Autodesk Inventor part; units mm, degrees
ref_plane "YZ Plane" through (0, 0, 0) normal (1, 0, 0) x (0, 1, 0)
ref_plane "XZ Plane" through (0, 0, 0) normal (0, 1, 0) x (-1, 0, 0)
ref_plane "XY Plane" through (0, 0, 0) normal (0, 0, 1) x (1, 0, 0)
sketch "Sketch2" plane through (0, 0, 0) normal (0, 0, 1) x (1, 0, 0)
  line L0 (0, 0) -> (87.9881, 0) construction
  line L1 (0, 0) -> (65.9905, 38.1011) construction
  line L2 (65.9905, 38.1011) -> (87.9881, 0) construction
  circle A0 centre (0, 0) radius 76.2 construction
  line L3 (62.5859, 43.4678) -> (34.9256, 27.4975)
  line L4 (68.9361, 32.4694) -> (41.2758, 16.4991)
  arc A1 (34.9256, 27.4975) -> (41.2758, 16.4991) centre (38.1007, 21.9983) ccw
  arc A2 (73.4536, 20.2735) -> (73.4536, -20.2735) centre (87.9881, 0) ccw
  arc A3 (73.4536, 20.2735) -> (68.9361, 32.4694) centre (0, 0) ccw
  line L5 (62.5873, -43.4657) -> (34.9265, -27.4963)
  arc A4 (41.2764, -16.4977) -> (34.9265, -27.4963) centre (38.1014, -21.997) ccw
  line L6 (68.9371, -32.4671) -> (41.2764, -16.4977)
  arc A5 (54.2842, -53.4759) -> (62.5873, -43.4657) centre (0, 0) ccw
  arc A6 (54.2842, -53.4759) -> (19.1694, -73.7494) centre (43.9941, -76.2) ccw
  line L7 (-6.3487, -75.9351) -> (-6.3493, -43.9954)
  arc A7 (6.3507, -43.9952) -> (-6.3493, -43.9954) centre (0.0007, -43.9953) ccw
  line L8 (6.3513, -75.9348) -> (6.3507, -43.9952)
  arc A8 (-19.1694, -73.7494) -> (-6.3487, -75.9351) centre (0, 0) ccw
  arc A9 (-19.1694, -73.7494) -> (-54.2842, -53.4759) centre (-43.9941, -76.2) ccw
  line L9 (-68.9361, -32.4694) -> (-41.2758, -16.4991)
  arc A10 (-34.9256, -27.4975) -> (-41.2758, -16.4991) centre (-38.1007, -21.9983) ccw
  line L10 (-62.5859, -43.4678) -> (-34.9256, -27.4975)
  arc A11 (-73.4536, -20.2735) -> (-68.9361, -32.4694) centre (0, 0) ccw
  arc A12 (-73.4536, -20.2735) -> (-73.4536, 20.2735) centre (-87.9881, 0) ccw
  line L11 (-62.5873, 43.4657) -> (-34.9265, 27.4963)
  arc A13 (-41.2764, 16.4977) -> (-34.9265, 27.4963) centre (-38.1014, 21.997) ccw
  line L12 (-68.9371, 32.4671) -> (-41.2764, 16.4977)
  arc A14 (-54.2842, 53.4759) -> (-62.5873, 43.4657) centre (0, 0) ccw
  arc A15 (-54.2842, 53.4759) -> (-19.1694, 73.7494) centre (-43.9941, 76.2) ccw
  line L13 (6.3487, 75.9351) -> (6.3493, 43.9954)
  arc A16 (-6.3507, 43.9952) -> (6.3493, 43.9954) centre (-0.0007, 43.9953) ccw
  line L14 (-6.3513, 75.9348) -> (-6.3507, 43.9952)
  arc A17 (19.1694, 73.7494) -> (6.3487, 75.9351) centre (0, 0) ccw
  arc A18 (19.1694, 73.7494) -> (54.2842, 53.4759) centre (43.9941, 76.2) ccw
  arc A19 (62.5859, 43.4678) -> (54.2842, 53.4759) centre (0, 0) ccw
  arc A20 (-6.3513, 75.9348) -> (-19.1694, 73.7494) centre (0, 0) ccw
  arc A21 (-68.9371, 32.4671) -> (-73.4536, 20.2735) centre (0, 0) ccw
  arc A22 (-62.5859, -43.4678) -> (-54.2842, -53.4759) centre (0, 0) ccw
  arc A23 (6.3513, -75.9348) -> (19.1694, -73.7494) centre (0, 0) ccw
  arc A24 (68.9371, -32.4671) -> (73.4536, -20.2735) centre (0, 0) ccw
  dimension "d6" = 87.9881
  dimension "d7" = 43.9953
  dimension "d8" = 76.2
  dimension "d9" = 12.7
  dimension "d10" = 32.2047
  dimension "d12" = 24.9453
  dimension "d15" = 360
extrude "Extrusion1" add sketch "Sketch2" along normal blind 16.9333
properties part number "Geneva Driven"
Verification items for the finished model (mm, model axes). A direction names the side the tool comes from. Round coordinates to 2 decimals unless told otherwise and drop trailing zeros. Order: outer loops, then holes, each group sorted by start corner. A loop starts at its lowest first (then second) coordinate and runs counter-clockwise, first axis right, second up.
1. Section check C-C on x = 48.5. Record the cut outline in (y, z).
Final values:
outline: (-51.66, 0) - (-35.33, 0) - (-35.33, 16.93) - (-51.66, 16.93) - close; (-20.67, 0) - (20.67, 0) - (20.67, 16.93) - (-20.67, 16.93) - close; (35.33, 0) - (51.66, 0) - (51.66, 16.93) - (35.33, 16.93) - close
2. Thickness scan on L1, parallel to Y at x = -55.5, z = 14; L2, parallel to Y at x = -34, z = 2; L3, parallel to X at y = -23, z = 6.5. Record the ranges inside material, lowest first.
Final values:
L1: y = -52.21 to -39.38, -24.71 to 24.71, 39.37 to 52.21
L2: y = -53.34 to -26.85, -17.15 to 17.15, 26.84 to 53.34
L3: x = -72.65 to -52.54, -31.83 to 31.83, 52.54 to 72.65
3. Access from +Z, -Z, +X, -X, +Y, -Y to the whole of each face (thin tool, end or side, straight path). Record for faces 5 (the cylindrical face through (-12.72, -75.13, 8.35)), 6 (the flat face through (-55.3, 24.594, 8.348)).
Final values:
face 5: +Z, -Z, -X, -Y
face 6: +Z, -Z
4. Section check A-A on x = -49.5. Record the cut outline in (y, z), then the cut area to 3 significant figures.
Final values:
outline: (-51.87, 0) - (-35.91, 0) - (-35.91, 16.93) - (-51.87, 16.93) - close; (-21.25, 0) - (21.25, 0) - (21.25, 16.93) - (-21.25, 16.93) - close; (35.91, 0) - (51.87, 0) - (51.87, 16.93) - (35.91, 16.93) - close
area: 1,260 mm2
5. Release check for a two-part mould opening along X. For faces 1 (the cylindrical face through (-58.708, 48.578, 8.348)), 2 (the cylindrical face through (71.424, 26.553, 8.348)), 3 (the flat face through (-1, 1, 16.933)), 4 (the cylindrical face through (-31.24, 54.76, 8.35)) record: +X half, -X half, draft (parallel to the pull), parting line (faces both ways), or undercut.
Final values:
face 1: -X half
face 2: +X half
face 3: draft
face 4: undercut
6. Section check B-B on y = -40. Record the cut outline in (x, z), then the cut area to 3 significant figures.
Final values:
outline: (-56.58, 0) - (-4.93, 0) - (-4.93, 16.93) - (-56.58, 16.93) - close; (4.94, 0) - (56.58, 0) - (56.58, 16.93) - (4.94, 16.93) - close
area: 1,750 mm2
7. Go/stop test with flat-tipped pins: P1, Ø1.5, axis at y = -38, z = 3, coming from the +X side; P2, Ø2, axis at y = 34, z = 8.5, coming from the +X side; P3, Ø8, axis at y = 27, z = 7, coming from the +X side; P4, Ø1.5, axis at x = -7, z = 8.5, coming from the +Y side. Record where each tip stops, or that it passes through.
Final values:
P1: stops at x = 54.42
P2: stops at x = 47.92
P3: stops at x = 72.65
P4: stops at y = 75.93
8. Section check D-D on x = 2. Record the cut outline in (y, z).
Final values:
outline: (-37.97, 0) - (37.97, 0) - (37.97, 16.93) - (-37.97, 16.93) - close
